Verification items for the finished model (mm, model axes). Face numbers are marked on the shaded views. A direction names the side the tool comes from. Give positions to 0.01 mm unless a question says otherwise; leave off trailing zeros. Order: outer loops, then holes, each group sorted by start corner. A loop starts at its lowest first (then second) coordinate and runs counter-clockwise, first axis right, second up. Notation, with made-up numbers: (34.5, 62) - (43.5, 62) arc R21 cw to (43.5, 86) - close; hole circle Ø10 at (69.25, 13). An arc over 180 degrees is marked (long way). Answer as a JSON object with one key per item and string values. Group by question number.
(1) Access from +Z, -Z, +X, -X, +Y, -Y to the whole of each face (thin tool, end or side, straight path). Record for the marked faces 5 and 6.
(2) Thickness scan on line 1 (Z direction, x = 0, y = 0.9); line 2 (Z direction, x = 0, y = 2.45); line 3 (Y direction, x = -4, z = 1.5). Record the ranges inside material, lowest first.
(3) Section check D-D (x = 4.5). Record the boundary of the cut face in (y, z).
(4) Section check C-C (z = -5.25). Record the boundary of the cut face in (x, y).
(5) Section check B-B (x = 0). Record the boundary of the cut face in (y, z).
(6) Mould release check, pull along Z, two halves, no side actions. Record for the marked faces 1, 2, 3 and 4: +Z half, -Z half, draft (parallel to the pull), parting line (faces both ways), or undercut.
(7) Section check A-A (z = 0). Record the boundary of the cut face in (x, y), then the cut area to 3 significant figures.
(8) Depth check by flat-ended pin: pin 1 Ø4 at (x, z) = (-4.5, 0) entering from +Y; pin 2 Ø2 at (x, y) = (-2.5, 12) entering from -Z; pin 3 Ø3.5 at (x, z) = (-0.5, 5.5) entering from +Y. Enter the tip coordinate at first touch or a pass-through.
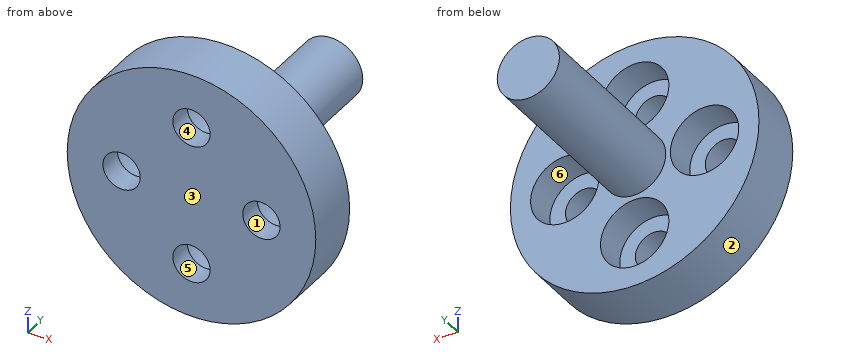
```python
from build123d import *

# Parameters (mm, degrees)
CBORE_FOR_M2_SHCS2_D           = 2.4
CBORE_FOR_M2_SHCS2_CBORE_D     = 4.4
CBORE_FOR_M2_SHCS2_CBORE_DEPTH = 2


with BuildPart() as part:
    # Sketch3 → Revolve1 (revolve)
    with BuildSketch(Plane.XY):
        Polygon((0, 0), (8, 0), (8, 3.5), (2, 3.5), (2, 14.5), (0, 14.5), align=None)
    revolve(axis=Axis((0, 14.5, 0), (0, -1, 0)))

    # CBORE for M2 SHCS2 (through all)
    with Locations(Plane(origin=(0, 3.5, 0), x_dir=(1, 0, 0), z_dir=(0, 1, 0))):
        with Locations((4.5, 0), (0, -4.5), (0, 4.5), (-4.5, 0)):
            CounterBoreHole(CBORE_FOR_M2_SHCS2_D / 2, CBORE_FOR_M2_SHCS2_CBORE_D / 2, CBORE_FOR_M2_SHCS2_CBORE_DEPTH)


solid = part.part
```
Solutions:
{
 "1": {"face 5": "+Y, -Y", "face 6": "+Y"},
 "2": {"line 1": "z = -8 to -5.7, -3.3 to 3.3, 5.7 to 8", "line 2": "z = -8 to -6.7, -2.3 to 2.3, 6.7 to 8", "line 3": "y = 0 to 1.5"},
 "3": {"outline": "(0, -6.61) - (3.5, -6.61) - (3.5, -2.2) - (1.5, -2.2) - (1.5, -1.2) - (0, -1.2) - close; (0, 1.2) - (1.5, 1.2) - (1.5, 2.2) - (3.5, 2.2) - (3.5, 6.61) - (0, 6.61) - close"},
 "4": {"outline": "(-6.04, 0) - (-0.94, 0) - (-0.94, 1.5) - (-2.07, 1.5) - (-2.07, 3.5) - (-6.04, 3.5) - close; (0.94, 0) - (6.04, 0) - (6.04, 3.5) - (2.07, 3.5) - (2.07, 1.5) - (0.94, 1.5) - close"},
 "5": {"outline": "(0, -8) - (3.5, -8) - (3.5, -6.7) - (1.5, -6.7) - (1.5, -5.7) - (0, -5.7) - close; (0, -3.3) - (1.5, -3.3) - (1.5, -2.3) - (3.5, -2.3) - (3.5, -2) - (14.5, -2) - (14.5, 2) - (3.5, 2) - (3.5, 2.3) - (1.5, 2.3) - (1.5, 3.3) - (0, 3.3) - close; (0, 5.7) - (1.5, 5.7) - (1.5, 6.7) - (3.5, 6.7) - (3.5, 8) - (0, 8) - close"},
 "6": {"face 1": "undercut", "face 2": "parting line", "face 3": "draft", "face 4": "undercut"},
 "7": {"outline": "(-8, 0) - (-5.7, 0) - (-5.7, 1.5) - (-6.7, 1.5) - (-6.7, 3.5) - (-8, 3.5) - close; (-3.3, 0) - (3.3, 0) - (3.3, 1.5) - (2.3, 1.5) - (2.3, 3.5) - (2, 3.5) - (2, 14.5) - (-2, 14.5) - (-2, 3.5) - (-2.3, 3.5) - (-2.3, 1.5) - (-3.3, 1.5) - close; (5.7, 0) - (8, 0) - (8, 3.5) - (6.7, 3.5) - (6.7, 1.5) - (5.7, 1.5) - close", "area": "75.2 mm2"},
 "8": {"pin 1": "stops at y = 1.5", "pin 2": "stops at z = -1.32", "pin 3": "stops at y = 3.5"}
}
